from build123d import *

# Parameters (mm, degrees)
F0_R     = 11.43
F0_R_2   = 5.08
F0_R_3   = 3.81
F1_DEPTH = 5.08


with BuildPart() as f1:
    # F0 (on Top) → F1 (new body)
    with BuildSketch(Plane.XY):
        with BuildLine():
            ThreePointArc((12.5445146004, -1.9812), (12.6610689799, -0.9936459568), (12.7, 0))
            ThreePointArc((12.7, 0), (12.6610689799, 0.9936459568), (12.5445146004, 1.9812))
            ThreePointArc((12.5445146004, 1.9812), (12.5436419256, 1.986717706), (12.5427668237, 1.9922350276))
            ThreePointArc((12.5427668237, 1.9922350276), (12.0784177569, 3.9245158286), (11.3183178852, 5.7607013678))
            ThreePointArc((11.3183178852, 5.7607013678), (11.3157828572, 5.7656793467), (11.3132456398, 5.77065621))
            ThreePointArc((11.3132456398, 5.77065621), (10.2745158286, 7.4648727041), (8.9842053561, 8.9763051485))
            ThreePointArc((8.9842053561, 8.9763051485), (8.9802561211, 8.9802561211), (8.9763051485, 8.9842053561))
            ThreePointArc((8.9763051485, 8.9842053561), (7.4648727041, 10.2745158286), (5.77065621, 11.3132456398))
            ThreePointArc((5.77065621, 11.3132456398), (5.7656793467, 11.3157828572), (5.7607013678, 11.3183178852))
            ThreePointArc((5.7607013678, 11.3183178852), (3.9245158286, 12.0784177569), (1.9922350276, 12.5427668237))
            ThreePointArc((1.9922350276, 12.5427668237), (1.986717706, 12.5436419256), (1.9812, 12.5445146004))
            ThreePointArc((1.9812, 12.5445146004), (0, 12.7), (-1.9812, 12.5445146004))
            ThreePointArc((-1.9812, 12.5445146004), (-1.986717706, 12.5436419256), (-1.9922350276, 12.5427668237))
            ThreePointArc((-1.9922350276, 12.5427668237), (-3.9245158286, 12.0784177569), (-5.7607013678, 11.3183178852))
            ThreePointArc((-5.7607013678, 11.3183178852), (-5.7656793467, 11.3157828572), (-5.77065621, 11.3132456398))
            ThreePointArc((-5.77065621, 11.3132456398), (-7.4648727041, 10.2745158286), (-8.9763051485, 8.9842053561))
            ThreePointArc((-8.9763051485, 8.9842053561), (-8.9802561211, 8.9802561211), (-8.9842053561, 8.9763051485))
            ThreePointArc((-8.9842053561, 8.9763051485), (-10.2745158286, 7.4648727041), (-11.3132456398, 5.77065621))
            ThreePointArc((-11.3132456398, 5.77065621), (-11.3157828572, 5.7656793467), (-11.3183178852, 5.7607013678))
            ThreePointArc((-11.3183178852, 5.7607013678), (-12.0784177569, 3.9245158286), (-12.5427668237, 1.9922350276))
            ThreePointArc((-12.5427668237, 1.9922350276), (-12.5436419256, 1.986717706), (-12.5445146004, 1.9812))
            Line((-12.5445146004, 1.9812), (-12.5445146004, 0))
            Line((-12.5445146004, 0), (-12.5445146004, -1.9812))
            ThreePointArc((-12.5445146004, -1.9812), (-12.5436419256, -1.986717706), (-12.5427668237, -1.9922350276))
            ThreePointArc((-12.5427668237, -1.9922350276), (-12.0784177569, -3.9245158286), (-11.3183178852, -5.7607013678))
            ThreePointArc((-11.3183178852, -5.7607013678), (-11.3157828572, -5.7656793467), (-11.3132456398, -5.77065621))
            ThreePointArc((-11.3132456398, -5.77065621), (-10.2745158286, -7.4648727041), (-8.9842053561, -8.9763051485))
            ThreePointArc((-8.9842053561, -8.9763051485), (-8.9802561211, -8.9802561211), (-8.9763051485, -8.9842053561))
            ThreePointArc((-8.9763051485, -8.9842053561), (-7.4648727041, -10.2745158286), (-5.77065621, -11.3132456398))
            ThreePointArc((-5.77065621, -11.3132456398), (-5.7656793467, -11.3157828572), (-5.7607013678, -11.3183178852))
            ThreePointArc((-5.7607013678, -11.3183178852), (-3.9245158286, -12.0784177569), (-1.9922350276, -12.5427668237))
            ThreePointArc((-1.9922350276, -12.5427668237), (-1.986717706, -12.5436419256), (-1.9812, -12.5445146004))
            ThreePointArc((-1.9812, -12.5445146004), (0, -12.7), (1.9812, -12.5445146004))
            ThreePointArc((1.9812, -12.5445146004), (1.986717706, -12.5436419256), (1.9922350276, -12.5427668237))
            ThreePointArc((1.9922350276, -12.5427668237), (3.9245158286, -12.0784177569), (5.7607013678, -11.3183178852))
            ThreePointArc((5.7607013678, -11.3183178852), (5.7656793467, -11.3157828572), (5.77065621, -11.3132456398))
            ThreePointArc((5.77065621, -11.3132456398), (7.4648727041, -10.2745158286), (8.9763051485, -8.9842053561))
            ThreePointArc((8.9763051485, -8.9842053561), (8.9802561211, -8.9802561211), (8.9842053561, -8.9763051485))
            ThreePointArc((8.9842053561, -8.9763051485), (10.2745158286, -7.4648727041), (11.3132456398, -5.77065621))
            ThreePointArc((11.3132456398, -5.77065621), (11.3157828572, -5.7656793467), (11.3183178852, -5.7607013678))
            ThreePointArc((11.3183178852, -5.7607013678), (12.0784177569, -3.9245158286), (12.5427668237, -1.9922350276))
            ThreePointArc((12.5427668237, -1.9922350276), (12.5436419256, -1.986717706), (12.5445146004, -1.9812))
        make_face()
        Circle(F0_R, mode=Mode.SUBTRACT)
        Circle(F0_R)
        Circle(F0_R_2, mode=Mode.SUBTRACT)
        Circle(F0_R_2)
        Circle(F0_R_3, mode=Mode.SUBTRACT)
        Circle(F0_R_3)
        with BuildLine():
            ThreePointArc((12.5445146004, 1.9812), (12.6610689799, 0.9936459568), (12.7, 0))
            ThreePointArc((12.7, 0), (12.6610689799, -0.9936459568), (12.5445146004, -1.9812))
            Line((12.5445146004, -1.9812), (16.5069146004, 0))
            Line((16.5069146004, 0), (12.5445146004, 1.9812))
        make_face()
        with BuildLine():
            ThreePointArc((11.3183178852, 5.7607013678), (12.0784177569, 3.9245158286), (12.5427668237, 1.9922350276))
            Line((12.5427668237, 1.9922350276), (15.6990086947, 5.1009171362))
            Line((15.6990086947, 5.1009171362), (11.3183178852, 5.7607013678))
        make_face()
        with BuildLine():
            Line((15.6990086947, -5.1009171362), (12.5427668237, -1.9922350276))
            ThreePointArc((12.5427668237, -1.9922350276), (12.0784177569, -3.9245158286), (11.3183178852, -5.7607013678))
            Line((11.3183178852, -5.7607013678), (15.6990086947, -5.1009171362))
        make_face()
        with BuildLine():
            ThreePointArc((8.9842053561, 8.9763051485), (10.2745158286, 7.4648727041), (11.3132456398, 5.77065621))
            Line((11.3132456398, 5.77065621), (13.3543744364, 9.702520963))
            Line((13.3543744364, 9.702520963), (8.9842053561, 8.9763051485))
        make_face()
        with BuildLine():
            Line((13.3543744364, -9.702520963), (11.3132456398, -5.77065621))
            ThreePointArc((11.3132456398, -5.77065621), (10.2745158286, -7.4648727041), (8.9842053561, -8.9763051485))
            Line((8.9842053561, -8.9763051485), (13.3543744364, -9.702520963))
        make_face()
        with BuildLine():
            ThreePointArc((5.77065621, 11.3132456398), (7.4648727041, 10.2745158286), (8.9763051485, 8.9842053561))
            Line((8.9763051485, 8.9842053561), (9.702520963, 13.3543744364))
            Line((9.702520963, 13.3543744364), (5.77065621, 11.3132456398))
        make_face()
        with BuildLine():
            Line((9.702520963, -13.3543744364), (8.9763051485, -8.9842053561))
            ThreePointArc((8.9763051485, -8.9842053561), (7.4648727041, -10.2745158286), (5.77065621, -11.3132456398))
            Line((5.77065621, -11.3132456398), (9.702520963, -13.3543744364))
        make_face()
        with BuildLine():
            ThreePointArc((1.9922350276, 12.5427668237), (3.9245158286, 12.0784177569), (5.7607013678, 11.3183178852))
            Line((5.7607013678, 11.3183178852), (5.1009171362, 15.6990086947))
            Line((5.1009171362, 15.6990086947), (1.9922350276, 12.5427668237))
        make_face()
        with BuildLine():
            Line((5.1009171362, -15.6990086947), (5.7607013678, -11.3183178852))
            ThreePointArc((5.7607013678, -11.3183178852), (3.9245158286, -12.0784177569), (1.9922350276, -12.5427668237))
            Line((1.9922350276, -12.5427668237), (5.1009171362, -15.6990086947))
        make_face()
        with BuildLine():
            ThreePointArc((-1.9812, 12.5445146004), (0, 12.7), (1.9812, 12.5445146004))
            Line((1.9812, 12.5445146004), (0, 16.5069146004))
            Line((0, 16.5069146004), (-1.9812, 12.5445146004))
        make_face()
        with BuildLine():
            Line((0, -16.5069146004), (1.9812, -12.5445146004))
            ThreePointArc((1.9812, -12.5445146004), (0, -12.7), (-1.9812, -12.5445146004))
            Line((-1.9812, -12.5445146004), (0, -16.5069146004))
        make_face()
        with BuildLine():
            ThreePointArc((-5.7607013678, 11.3183178852), (-3.9245158286, 12.0784177569), (-1.9922350276, 12.5427668237))
            Line((-1.9922350276, 12.5427668237), (-5.1009171362, 15.6990086947))
            Line((-5.1009171362, 15.6990086947), (-5.7607013678, 11.3183178852))
        make_face()
        with BuildLine():
            Line((-5.1009171362, -15.6990086947), (-1.9922350276, -12.5427668237))
            ThreePointArc((-1.9922350276, -12.5427668237), (-3.9245158286, -12.0784177569), (-5.7607013678, -11.3183178852))
            Line((-5.7607013678, -11.3183178852), (-5.1009171362, -15.6990086947))
        make_face()
        with BuildLine():
            ThreePointArc((-8.9763051485, 8.9842053561), (-7.4648727041, 10.2745158286), (-5.77065621, 11.3132456398))
            Line((-5.77065621, 11.3132456398), (-9.702520963, 13.3543744364))
            Line((-9.702520963, 13.3543744364), (-8.9763051485, 8.9842053561))
        make_face()
        with BuildLine():
            Line((-9.702520963, -13.3543744364), (-5.77065621, -11.3132456398))
            ThreePointArc((-5.77065621, -11.3132456398), (-7.4648727041, -10.2745158286), (-8.9763051485, -8.9842053561))
            Line((-8.9763051485, -8.9842053561), (-9.702520963, -13.3543744364))
        make_face()
        with BuildLine():
            ThreePointArc((-11.3132456398, 5.77065621), (-10.2745158286, 7.4648727041), (-8.9842053561, 8.9763051485))
            Line((-8.9842053561, 8.9763051485), (-13.3543744364, 9.702520963))
            Line((-13.3543744364, 9.702520963), (-11.3132456398, 5.77065621))
        make_face()
        with BuildLine():
            Line((-13.3543744364, -9.702520963), (-8.9842053561, -8.9763051485))
            ThreePointArc((-8.9842053561, -8.9763051485), (-10.2745158286, -7.4648727041), (-11.3132456398, -5.77065621))
            Line((-11.3132456398, -5.77065621), (-13.3543744364, -9.702520963))
        make_face()
        with BuildLine():
            ThreePointArc((-12.5427668237, 1.9922350276), (-12.0784177569, 3.9245158286), (-11.3183178852, 5.7607013678))
            Line((-11.3183178852, 5.7607013678), (-15.6990086947, 5.1009171362))
            Line((-15.6990086947, 5.1009171362), (-12.5427668237, 1.9922350276))
        make_face()
        with BuildLine():
            Line((-15.6990086947, -5.1009171362), (-11.3183178852, -5.7607013678))
            ThreePointArc((-11.3183178852, -5.7607013678), (-12.0784177569, -3.9245158286), (-12.5427668237, -1.9922350276))
            Line((-12.5427668237, -1.9922350276), (-15.6990086947, -5.1009171362))
        make_face()
        with BuildLine():
            ThreePointArc((-12.7, 0), (-12.6610689799, 0.9936459568), (-12.5445146004, 1.9812))
            Line((-12.5445146004, 1.9812), (-16.5069146004, 0))
            Line((-16.5069146004, 0), (-12.7, 0))
        make_face()
        with BuildLine():
            Line((-16.5069146004, 0), (-12.5445146004, -1.9812))
            ThreePointArc((-12.5445146004, -1.9812), (-12.6610689799, -0.9936459568), (-12.7, 0))
            Line((-12.7, 0), (-16.5069146004, 0))
        make_face()
        with BuildLine():
            Line((-12.5445146004, 0), (-12.5445146004, 1.9812))
            ThreePointArc((-12.5445146004, 1.9812), (-12.6610689799, 0.9936459568), (-12.7, 0))
            Line((-12.7, 0), (-12.5445146004, 0))
        make_face()
        with BuildLine():
            ThreePointArc((-12.7, 0), (-12.6610689799, -0.9936459568), (-12.5445146004, -1.9812))
            Line((-12.5445146004, -1.9812), (-12.5445146004, 0))
            Line((-12.5445146004, 0), (-12.7, 0))
        make_face()
    extrude(amount=F1_DEPTH)


solid = f1.part
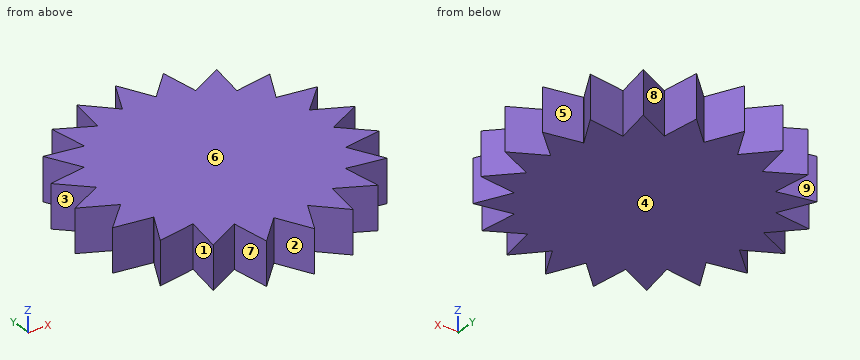
Could you check a few things on this model? Use its own coordinates, in mm. Face numbers are marked on the shaded views. A direction names the side the tool comes from. Coordinates: 2 decimals unless noted, no trailing zeros. Loops run counter-clockwise (first coordinate to the right, second up) from the corner with the lowest first, then second, coordinate; pieces in that order, holes last.
1. I need wall thicknesses on L1, parallel to Y at x = 14, z = 1.3; L2, parallel to Y at x = 15.5, z = 2.05; L3, parallel to Y at x = 13, z = 3.8. Which ranges of each line are inside material? Lowest first, please.
2. For the marked faces 1, 2, 3, 4 and 5, which set-ups out of +Z, -Z, +X, -X, +Y, -Y let a thin tool reach every point of the face, with its end or its side?
3. Imagine slicing it at C-C (y = -3). Please give me the cut outline in (x, z).
4. We'd pull the mould along Y, two halves only. Please class the marked faces 6, 7, 8 and 9: released by +Y, released by -Y, zero draft, split by the parting line, or undercut.
5. Imagine slicing it at B-B (x = 1). Please give me the cut outline in (y, z), and give its area (3 significant figures).
6. Imagine slicing it at A-A (x = -14). Please give me the cut outline in (y, z).
7. For P1, Ø5, axis at x = 3, y = -6.5, coming from the -Z side; P2, Ø2, axis at x = -5, z = 2.5, coming from the +Y side; P3, Ø1.5, axis at y = -4, z = 3, coming from the +X side, each with a flat end and sliding along its axis, tell me the tip position at first contact or that it passes through.
Computed values:
1. L1: y = -5.36 to -3.43, -1.25 to 1.25, 3.43 to 5.36
1. L2: y = -5.13 to -4.9, -0.5 to 0.5, 4.9 to 5.13
1. L3: y = -9.64 to -9.02, -5.51 to -2.44, -1.75 to 1.75, 2.44 to 5.51, 9.02 to 9.64
2. face 1: +Z, -Z
2. face 2: +Z, -Z, -Y
2. face 3: +Z, -Z, -X
2. face 4: -Z, +X, -X, +Y, -Y
2. face 5: +Z, -Z, +X
3. outline: (-13.57, 0) - (13.57, 0) - (13.57, 5.08) - (-13.57, 5.08) - close
4. face 6: zero draft
4. face 7: released by -Y
4. face 8: released by +Y
4. face 9: undercut
5. outline: (-14.51, 0) - (14.51, 0) - (14.51, 5.08) - (-14.51, 5.08) - close
5. area: 147 mm2
6. outline: (-5.36, 0) - (-3.43, 0) - (-3.43, 5.08) - (-5.36, 5.08) - close; (-1.25, 0) - (1.25, 0) - (1.25, 5.08) - (-1.25, 5.08) - close; (3.43, 0) - (5.36, 0) - (5.36, 5.08) - (3.43, 5.08) - close
7. P1: stops at z = 0
7. P2: stops at y = 15.7
7. P3: stops at x = 15.34
